Could you check a few things on this drawing? It's one solid part, dimensions in mm from its lowest x, y, z. A direction names the side the tool comes from. Give positions to 0.01 mm unless a question says otherwise; leave off trailing zeros. Order: outer loops, then holes, each group sorted by start corner. A loop starts at its lowest first (then second) coordinate and runs counter-clockwise, first axis right, second up. Notation, with made-up numbers: M 33.25,-13 L 69.25,-13 A10 cw 69.25,1 Z; hole C -13.5,2 d5. An arc over 180 degrees is marked long. Use one line per item in the form item = value.
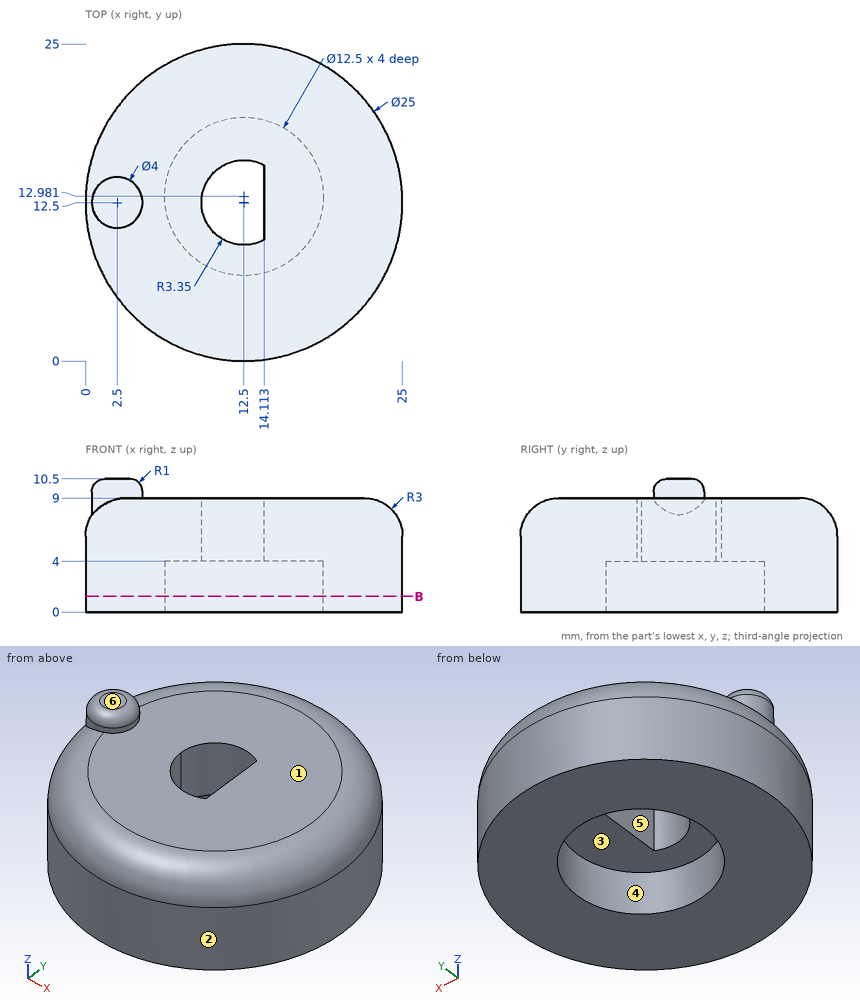
Q1. I want a section at B-B on z = 1.25. Write out the boundary of the cut face in (x, y), then the cut area to 3 significant figures.
Found:
outline = C 12.5,12.5 d25; hole C 12.5,12.98 d12.5
area = 368 mm²
Q2. I need wall thicknesses on L1, parallel to Y at x = 12.5, z = 1.75; L2, parallel to Z at x = 18, y = 9.5; L3, parallel to X at y = 18.5, z = 2.75 (1 decimal). Which ranges of each line are inside material? Lowest first, please.
Found:
L1 = 0 to 6.73, 19.23 to 25
L2 = 0 to 9
L3 = 1.5 to 9.6, 15.4 to 23.5
Q3. I'm going to push flat-ended pins straight in: pin 1 Ø4 at (x, z) = (7, 5.5) entering from -Y; pin 2 Ø4 at (y, z) = (19, 5.5) entering from +X; pin 3 Ø7.5 at (x, y) = (12.5, 12.98) entering from -Z. Where does each tip first touch, or does it pass through?
Found:
pin_1 = 0.5
pin_2 = 24.16
pin_3 = 4
Q4. On a 3-axis mill with a long thin cutter (end or side, diameter ignored), from which of +Z, -Z, +X, -X, +Y, -Y can I reach the whole of each face in a straight line? I mean the marked faces 5 and 6. Say none if no direction works.
Found:
face_5 = +Z, -Z
face_6 = +Z, +X, -X, +Y, -Y
Q5. Thinking about a two-plate mould opening in Y: for the marked faces 1, 2, 3 and 4, which applies, +Y half, -Y half, draft (parallel to the pull), parting line (faces both ways), or undercut?
Found:
face_1 = draft
face_2 = parting line
face_3 = undercut
face_4 = undercut
